Here's how the part is built. I have some questions about the finished solid (model axes, mm). A direction names the side the tool comes from. Give positions to 0.01 mm unless a question says otherwise; leave off trailing zeros. Order: outer loops, then holes, each group sorted by start corner. A loop starts at its lowest first (then second) coordinate and runs counter-clockwise, first axis right, second up. Notation, with made-up numbers: M 11,81.25 L 26,81.25 A30 ccw 26,119.25 Z; hole C 78.5,12 d4. An arc over 180 degrees is marked long. One line per item, written item: value. Start each with the question number.
from build123d import *

# Parameters (mm, degrees)
F0_W     = 77.51
F0_H     = 77.519
F0_R     = 4
F0_R_2   = 5
F0_R_3   = 2.55
F1_DEPTH = 10
F2_R     = 5
F3_DEPTH = 4


# Not quite as in the source:
# - a feature names something its author has since deleted; it is built from what else it names


with BuildPart() as f1:
    # F0 (on Top) → F1 (new body)
    with BuildSketch(Plane.XY):
        Rectangle(F0_W, F0_H)
        with Locations((-30, -29.9995)):
            Circle(F0_R, mode=Mode.SUBTRACT)
        with Locations((-20, -19.9995)):
            Circle(F0_R_2, mode=Mode.SUBTRACT)
        with Locations((30, -29.9995)):
            Circle(F0_R, mode=Mode.SUBTRACT)
        with Locations((20, -19.9995)):
            Circle(F0_R_2, mode=Mode.SUBTRACT)
        with Locations((-20, 19.9995)):
            Circle(F0_R_2, mode=Mode.SUBTRACT)
        with Locations((-30, 29.9995)):
            Circle(F0_R, mode=Mode.SUBTRACT)
        with Locations((20, 19.9995)):
            Circle(F0_R_2, mode=Mode.SUBTRACT)
        with Locations((30, 29.9995)):
            Circle(F0_R, mode=Mode.SUBTRACT)
        with Locations((-20, 19.9995)):
            Circle(F0_R_2)
        with Locations((-20, 19.9995)):
            Circle(F0_R_3, mode=Mode.SUBTRACT)
        with Locations((20, 19.9995)):
            Circle(F0_R_2)
        with Locations((20, 19.9995)):
            Circle(F0_R_3, mode=Mode.SUBTRACT)
        with Locations((20, -19.9995)):
            Circle(F0_R_2)
        with Locations((20, -19.9995)):
            Circle(F0_R_3, mode=Mode.SUBTRACT)
        with Locations((-20, -19.9995)):
            Circle(F0_R_2)
        with Locations((-20, -19.9995)):
            Circle(F0_R_3, mode=Mode.SUBTRACT)
    extrude(amount=F1_DEPTH)

    # F2
    f2_edges = [f1.edges().sort_by_distance(p)[0] for p in [
        (38.755, -38.7595, 5),
        (-38.755, -38.7595, 5),
        (38.755, 38.7595, 5),
        (-38.755, 38.7595, 5),
    ]]
    fillet(f2_edges, radius=F2_R)

    # F0 (on Top) → F3 (cut)
    with BuildSketch(Plane.XY):
        with Locations((-20, 19.9995)):
            Circle(F0_R_2)
        with Locations((-20, 19.9995)):
            Circle(F0_R_3, mode=Mode.SUBTRACT)
        with Locations((20, 19.9995)):
            Circle(F0_R_2)
        with Locations((20, 19.9995)):
            Circle(F0_R_3, mode=Mode.SUBTRACT)
        with Locations((-20, -19.9995)):
            Circle(F0_R_2)
        with Locations((-20, -19.9995)):
            Circle(F0_R_3, mode=Mode.SUBTRACT)
        with Locations((20, -19.9995)):
            Circle(F0_R_2)
        with Locations((20, -19.9995)):
            Circle(F0_R_3, mode=Mode.SUBTRACT)
    extrude(amount=F3_DEPTH, mode=Mode.SUBTRACT)


solid = f1.part
Item 1: For faces 4 (the face through (-38.755, 0, 5)), 5 (the face through (-24, 23, 2)), which set-ups out of +Z, -Z, +X, -X, +Y, -Y let a thin tool reach every point of the face, with its end or its side?
Item 2: I want a section at C-C on z = 5.75. Count the separate pieces of the cut face and the enclosed holes in it, plus the area to 3 significant figures.
Item 3: We'd pull the mould along X, two halves only. Please class faces 1 (the face through (38.755, 0, 5)), 2 (the face through (-1, 1, 10)), 3 (the face through (-24, -17, 2)): +X half, -X half, draft (parallel to the pull), parting line (faces both ways), or undercut.
Item 4: I want a section at A-A on x = -20. Write out the boundary of the cut face in (y, z).
Item 5: Please list where these lines run through material, in increasing order: probe 1 along Y at (x, z) = (20, 1.75); probe 2 along Y at (x, z) = (20, 6.5); probe 3 along X at (y, z) = (20, 1) (3 decimals). Write a range as [from, to].
Item 6: I want a section at D-D on x = 30. Write out the boundary of the cut face in (y, z).
Item 7: Will these pins go through, and if not, where does the flat tip stop? P1, Ø9, axis at x = 30, y = -30, coming from the -Z side; P2, Ø5, axis at x = 21, y = -21, coming from the -Z side; P3, Ø4.5, axis at x = -20, y = -20, coming from the -Z side.
Item 8: I want a section at B-B on y = -21. Write out the boundary of the cut face in (x, z) (3 decimals).
Answer below:
1. face 4: +Z, -Z, -X, +Y, -Y
1. face 5: -Z
2. separate pieces: 1
2. enclosed holes: 8
2. area: 5,700 mm²
3. face 1: +X half
3. face 2: draft
3. face 3: undercut
4. outline: M -38.76,0 L -25,0 L -25,4 L -22.55,4 L -22.55,10 L -38.76,10 Z; M -17.45,4 L -15,4 L -15,0 L 15,0 L 15,4 L 17.45,4 L 17.45,10 L -17.45,10 Z; M 22.55,4 L 25,4 L 25,0 L 38.76,0 L 38.76,10 L 22.55,10 Z
5. probe 1: y = [-38.76, -25], [-15, 15], [25, 38.76]
5. probe 2: y = [-38.76, -22.55], [-17.45, 17.45], [22.55, 38.76]
5. probe 3: x = [-38.755, -25], [-15, 15], [25, 38.755]
6. outline: M -38.76,0 L -34,0 L -34,10 L -38.76,10 Z; M -26,0 L 26,0 L 26,10 L -26,10 Z; M 34,0 L 38.76,0 L 38.76,10 L 34,10 Z
7. P1: stops at z = 0
7. P2: stops at z = 4
7. P3: passes through
8. outline: M -38.755,0 L -24.899,0 L -24.899,4 L -22.346,4 L -22.346,10 L -38.755,10 Z; M -17.654,4 L -15.101,4 L -15.101,0 L 15.101,0 L 15.101,4 L 17.654,4 L 17.654,10 L -17.654,10 Z; M 22.346,4 L 24.899,4 L 24.899,0 L 38.755,0 L 38.755,10 L 22.346,10 Z
